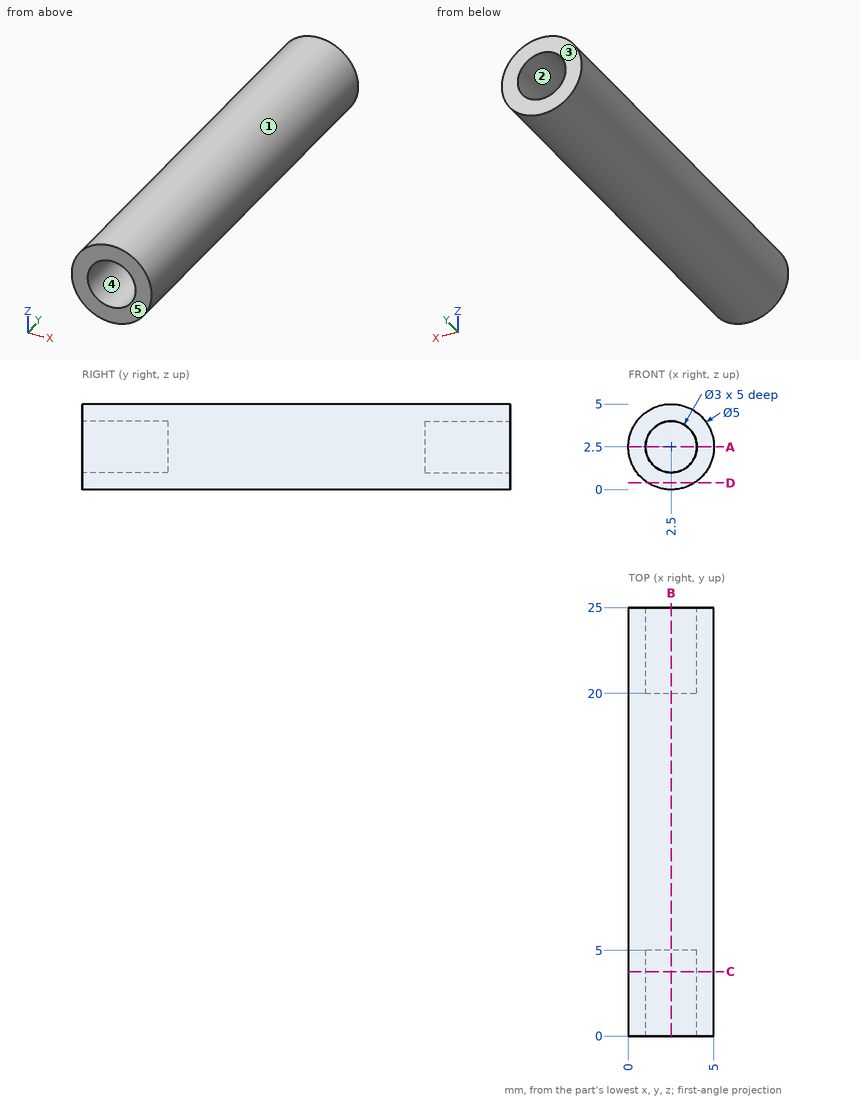
Can you work these out from the drawing? Everything is in mm from the part's minimum corner. A direction names the side the tool comes from. Give positions to 0.01 mm unless a question says otherwise; leave off trailing zeros. Order: outer loops, then holes, each group sorted by start corner. A loop starts at its lowest first (then second) coordinate and runs counter-clockwise, first axis right, second up. Notation, with made-up numbers: (-30, 38.5) -> (-24, 38.5) arc R22 ccw to (-24, 73.5) -> close; hole circle Ø3 at (-37.75, 79.25). An arc over 180 degrees is marked (long way). Return JSON: item names as keys, results as strings.
1. Imagine slicing it at D-D on z = 0.4. List the corners of the cut face in (x, y) for me.
Answer list:
{"outline": "(1.14, 0) -> (3.86, 0) -> (3.86, 25) -> (1.14, 25) -> close"}
2. For pin 1 Ø2 at (x, y) = (0.5, 3) entering from -Z; pin 2 Ø1.5 at (x, z) = (2, 2) entering from +Y; pin 3 Ø0.9 at (x, z) = (3, 3) entering from -Y, each with a flat end and sliding along its axis, tell me the tip position at first contact or that it passes through.
Answer list:
{"pin 1": "stops at z = 0.21", "pin 2": "stops at y = 20", "pin 3": "stops at y = 5"}
3. Thinking about a two-plate mould opening in X: for the marked faces 1, 2 and 3, which applies, pulls with the +X half, pulls with the -X half, needs draft (parallel to the pull), parting line crosses it, or undercut?
Answer list:
{"face 1": "parting line crosses it", "face 2": "undercut", "face 3": "needs draft"}
4. On a 3-axis mill with a long thin cutter (end or side, diameter ignored), from which of +Z, -Z, +X, -X, +Y, -Y can I reach the whole of each face in a straight line? I mean the marked faces 4 and 5. Say none if no direction works.
Answer list:
{"face 4": "-Y", "face 5": "+Z, -Z, +X, -X, -Y"}
5. Imagine slicing it at C-C on y = 3.75. List the corners of the cut face in (x, z) for me.
Answer list:
{"outline": "circle Ø5 at (2.5, 2.5); hole circle Ø3 at (2.5, 2.5)"}
6. I need wall thicknesses on line 1 (Z direction, x = 2.5, y = 2.75); line 2 (Y direction, x = 2.8, z = 2.1); line 3 (X direction, y = 18.5, z = 4.2). Which ranges of each line are inside material? Lowest first, please. Write a range as from..to.
Answer list:
{"line 1": "z = 0..1, 4..5", "line 2": "y = 5..20", "line 3": "x = 0.67..4.33"}
7. Imagine slicing it at A-A on z = 2.5. List the corners of the cut face in (x, y) for me, then the cut area to 3 significant figures.
Answer list:
{"outline": "(0, 0) -> (1, 0) -> (1, 5) -> (4, 5) -> (4, 0) -> (5, 0) -> (5, 25) -> (4, 25) -> (4, 20) -> (1, 20) -> (1, 25) -> (0, 25) -> close", "area": "95.0 mm2"}
8. Imagine slicing it at B-B on x = 2.5. List the corners of the cut face in (y, z) for me.
Answer list:
{"outline": "(0, 0) -> (25, 0) -> (25, 1) -> (20, 1) -> (20, 4) -> (25, 4) -> (25, 5) -> (0, 5) -> (0, 4) -> (5, 4) -> (5, 1) -> (0, 1) -> close"}
